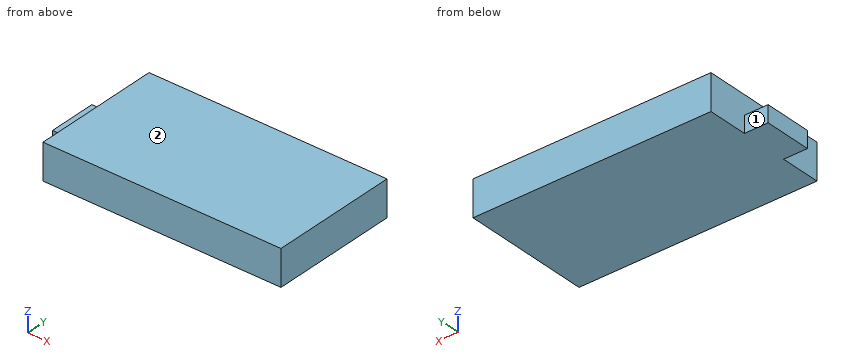
```python
from build123d import *

# Parameters (mm, degrees)
SKETCH1_W           = 50
SKETCH1_H           = 27
BOSS_EXTRUDE1_DEPTH = 7.5
SKETCH2_W           = 3.5
SKETCH2_H           = 10
BOSS_EXTRUDE2_DEPTH = 5


with BuildPart() as part:
    # Sketch1 → Boss-Extrude1 (new body)
    with BuildSketch(Plane.XY):
        Rectangle(SKETCH1_W, SKETCH1_H)
    extrude(amount=BOSS_EXTRUDE1_DEPTH)

    # Sketch2 → Boss-Extrude2 (add)
    with BuildSketch(Plane.ZY.offset(25)):
        with Locations((1.75, 0)):
            Rectangle(SKETCH2_W, SKETCH2_H)
    extrude(amount=BOSS_EXTRUDE2_DEPTH)


solid = part.part
```
Check sheet for the modelled part. Datum: model origin and axes. Units: mm. Face numbers are marked on the shaded views. A direction names the side the tool comes from. Round coordinates to 2 decimals unless told otherwise and drop trailing zeros. Loops run counter-clockwise (first coordinate to the right, second up) from the corner with the lowest first, then second, coordinate; pieces in that order, holes last. Notation, with made-up numbers: (0, 62) -> (25, 62) arc R10 cw to (25, 81) -> close; hole circle Ø5 at (-37.5, 83.5). An arc over 180 degrees is marked (long way). Write item = value, one per line. Start each with the question number.
1) Sectioned sample at A-A, the plane z = 1.75. Record the cut outline in (x, y), plus the area to 3 significant figures.
2) Thickness scan on probe 1 along X at (y, z) = (-2.5, 4.75). Record the ranges inside material, lowest first.
3) Sectioned sample at B-B, the plane y = -3. Record the cut outline in (x, z).
4) Sectioned sample at C-C, the plane x = -25.5. Record the cut outline in (y, z).
5) Sectioned sample at D-D, the plane z = 6. Record the cut outline in (x, y).
6) Set-up check for the marked faces 1 and 2: record each of +Z, -Z, +X, -X, +Y, -Y from which the full face is reachable in a straight line by a thin tool's end or side.
7) Gauge pin test, flat ends, axial feed: pin 1 Ø1.5 at (x, y) = (-27, -2) entering from +Z; pin 2 Ø1.8 at (x, z) = (-26.5, 1) entering from +Y; pin 3 Ø1 at (x, z) = (-26.5, 1) entering from -Y. Record the tip position at first contact, or that the pin passes through.
Results are:
q1.outline = (-30, -5) -> (-25, -5) -> (-25, -13.5) -> (25, -13.5) -> (25, 13.5) -> (-25, 13.5) -> (-25, 5) -> (-30, 5) -> close
q1.area = 1,400 mm^2
q2.probe_1 = -25 to 25
q3.outline = (-30, 0) -> (25, 0) -> (25, 7.5) -> (-25, 7.5) -> (-25, 3.5) -> (-30, 3.5) -> close
q4.outline = (-5, 0) -> (5, 0) -> (5, 3.5) -> (-5, 3.5) -> close
q5.outline = (-25, -13.5) -> (25, -13.5) -> (25, 13.5) -> (-25, 13.5) -> close
q6.face_1 = +Z, -Z, -X, +Y
q6.face_2 = +Z, +X, -X, +Y, -Y
q7.pin_1 = 3.5
q7.pin_2 = 5
q7.pin_3 = -5
